Read the model definition and answer for the solid it produces. Units are mm, in the model's axes. A direction names the side the tool comes from. Give positions to 0.01 mm unless a question says otherwise; leave off trailing zeros. Write each loop counter-clockwise with the first axis right and the second up, starting at its lowest first coordinate (ties: lowest second). Pieces come first, ordered by that corner, then holes. Notation, with made-up numbers: (-14.75, -10) -> (31.25, -10) arc R23 cw to (31.25, 22) -> close; hole circle Ø5 at (74, 68.5). An arc over 180 degrees is marked (long way). Put each result on its own line as item: value. Start each with the question number.
Solid Edge part; units mm, degrees
sketch "Sketch1" plane through (0, 0, 0) normal (0, 0, 1) x (1, 0, 0)
  circle A0 centre (0, 0) radius 59.65
extrude "Protrusion1" add sketch "Sketch1" against normal blind 25
sketch "Sketch2" plane through (0, 0, 0) normal (0, 0, 1) x (1, 0, 0)
  circle A0 centre (31.55, 31.55) radius 2.65
  circle A1 centre (-31.55, 31.55) radius 2.65
  circle A2 centre (31.55, -31.55) radius 2.65
  circle A3 centre (-31.55, -31.55) radius 2.65
extrude "ExtrudedCutout_2" cut sketch "Sketch2" against normal blind 25
sketch "Sketch3" plane through (0, 0, 0) normal (0, 0, 1) x (1, 0, 0)
  line L0 (-31.35, -31.525) -> (31.35, -31.525)
  line L1 (31.35, -31.525) -> (31.35, 31.525)
  line L2 (31.35, 31.525) -> (-31.35, 31.525)
  line L3 (-31.35, 31.525) -> (-31.35, -31.525)
extrude "ExtrudedCutout_7" cut sketch "Sketch3" against normal blind 25
1) For a pull along Y with two mould halves and no side action, classify faces 3 (the face through (-1, -39, -25)), 4 (the face through (31.35, 0, -12)), 5 (the face through (56.9, 17.9, -12.3)) as pulls with the +Y half, pulls with the -Y half, needs draft (parallel to the pull), parting line crosses it, or undercut.
2) A cutting plane is placed at B-B on y = 0. Give the vertices of the cut face in (x, z), and give its area (4 significant figures).
3) Each of these flat-tipped pins is pushed along its axis until it touches: pin 1 Ø6 at (x, z) = (20.5, -22) entering from +Y; pin 2 Ø1.5 at (y, z) = (3, -16) entering from +X; pin 3 Ø8 at (y, z) = (29, -18) entering from -X; pin 4 Ø1 at (x, y) = (-17, 36) entering from +Z. Where does it stop, or does it pass through?
4) Straight lines are drawn through the part: line 1 (Y direction, x = -1, z = -12.5) (3 decimals); line 2 (Y direction, x = 31.55, z = -15); line 3 (X direction, y = 0.5, z = -5.75). For each, find the intervals that lie inside material, in ascending order. Write a range as [from, to].
5) A cutting plane is placed at C-C on x = -7. Give the vertices of the cut face in (y, z) (3 decimals), and give its area (3 significant figures).
6) A cutting plane is placed at A-A on z = -20.5. Give the vertices of the cut face in (x, y) (3 decimals).
7) For faces 1 (the face through (-1, -39, 0)), 2 (the face through (0, -31.525, -12)), determine the directions among +Z, -Z, +X, -X, +Y, -Y from which every point of the face is accessible in a straight line to the end or side of a thin tool.
8) A cutting plane is placed at D-D on x = 36.5. Give the vertices of the cut face in (y, z), and give its area (3 significant figures).
Results found:
1. face 3: needs draft
1. face 4: undercut
1. face 5: parting line crosses it
2. outline: (-59.65, -25) -> (-31.35, -25) -> (-31.35, 0) -> (-59.65, 0) -> close; (31.35, -25) -> (59.65, -25) -> (59.65, 0) -> (31.35, 0) -> close
2. area: 1,415 mm²
3. pin 1: stops at y = 57.03
3. pin 2: stops at x = 59.61
3. pin 3: stops at x = -54.16
3. pin 4: stops at z = 0
4. line 1: y = [-59.642, -31.525], [31.525, 59.642]
4. line 2: y = [-50.62, -34.2], [-28.9, 28.9], [34.2, 50.62]
4. line 3: x = [-59.65, -31.35], [31.35, 59.65]
5. outline: (-59.238, -25) -> (-31.525, -25) -> (-31.525, 0) -> (-59.238, 0) -> close; (31.525, -25) -> (59.238, -25) -> (59.238, 0) -> (31.525, 0) -> close
5. area: 1,390 mm²
6. outline: circle Ø119.3 at (0, 0); hole (-31.35, -28.908) arc R2.65 ccw (long way) to (-28.9, -31.525) -> (28.9, -31.525) arc R2.65 ccw (long way) to (31.35, -28.908) -> (31.35, 28.908) arc R2.65 ccw (long way) to (28.9, 31.525) -> (-28.9, 31.525) arc R2.65 ccw (long way) to (-31.35, 28.908) -> close
7. face 1: +Z, +X, -X, +Y, -Y
7. face 2: +Z, -Z
8. outline: (-47.18, -25) -> (47.18, -25) -> (47.18, 0) -> (-47.18, 0) -> close
8. area: 2,360 mm²
